Autodesk Inventor part; units mm, degrees
ref_plane "YZ Plane" through (0, 0, 0) normal (1, 0, 0) x (0, 1, 0)
ref_plane "XZ Plane" through (0, 0, 0) normal (0, 1, 0) x (-1, 0, 0)
ref_plane "XY Plane" through (0, 0, 0) normal (0, 0, 1) x (1, 0, 0)
sketch "Sketch1" plane through (0, 0, 0) normal (1, 0, 0) x (0, 1, 0)
  line L0 (-26.75, 11.75) -> (26.75, 11.75)
  line L1 (26.75, 11.75) -> (26.75, -11.75)
  line L2 (26.75, -11.75) -> (-26.75, -11.75)
  line L3 (-26.75, -11.75) -> (-26.75, 11.75)
  line L4 (-26.75, 11.75) -> (26.75, -11.75) construction
  line L5 (26.75, 11.75) -> (-26.75, -11.75) construction
  circle A0 centre (16.75, 0) radius 2.75
  circle A1 centre (-16.75, 0) radius 2.75
  point P0 (0, 0)
  dimension "d0" = 53.5
  dimension "d1" = 23.5
  dimension "d2" = 5.5
  dimension "d3" = 5.5
  dimension "d4" = 10
  dimension "d5" = 10
  dimension "d6" = 11.75
  dimension "d7" = 11.75
extrude "Extrusion1" add sketch "Sketch1" along normal blind 5
sketch "Sketch2" plane through (5, 0, 0) normal (1, 0, 0) x (0, 0, -1)
  line L0 (-11.75, 26.75) -> (-11.75, -26.75)
  line L1 (-11.75, 26.75) -> (11.75, 26.75)
  line L2 (11.75, 26.75) -> (11.75, 21.75)
  line L3 (11.75, 21.75) -> (-11.75, 21.75)
  line L4 (-11.75, 21.75) -> (-11.75, 26.75)
  line L5 (-11.75, -26.75) -> (11.75, -26.75)
  line L6 (-11.75, -26.75) -> (11.75, -26.75)
  line L7 (11.75, -26.75) -> (11.75, -21.75)
  line L8 (11.75, -21.75) -> (-11.75, -21.75)
  line L9 (-11.75, -21.75) -> (-11.75, -26.75)
  point P0 (0, 0)
  dimension "d10" = 23.5
  dimension "d11" = 5
  dimension "d12" = 23.5
  dimension "d13" = 5
extrude "Extrusion2" add sketch "Sketch2" along normal blind 15
sketch "Sketch3" plane through (0, 26.75, 11.75) normal (0, 1, 0) x (1, 0, 0)
  circle A0 centre (10, 11.75) radius 2.75
  line L0 (0, 0) -> (0, 23.5)
  line L1 (0, 0) -> (20, 0)
  point P0 (0, 11.75)
  dimension "d16" = 5.5
  dimension "d17" = 10
  dimension "d18" = 11.75
extrude "Extrusion3" cut sketch "Sketch3" against normal up to surface (53.5 mm away)
properties part number "Extrusion ends" material "Aluminum 6061"
Source: CAD feature listing. Evaluate the final solid. Frame: model axes, mm. A direction names the side the tool comes from. Round coordinates to 2 decimals unless told otherwise and drop trailing zeros. Loops run counter-clockwise (first coordinate to the right, second up) from the corner with the lowest first, then second, coordinate; pieces in that order, holes last.
1. Access query for faces 1 (the flat face through (0, 0, 0)), 2 (the flat face through (5, 0, 0)). Directions: +Z, -Z, +X, -X, +Y, -Y. A direction counts if a zero-diameter tool reaches every point of the face in a straight line with its end or side. Return the directions, or none.
2. Ray query, L1, parallel to Y at x = 13.5, z = 6.75; L2, parallel to Z at x = 10, y = -24.65; L3, parallel to X at y = 2, z = -2. Return the intervals inside material, ascending.
3. Section query B-B on y = 16.75. Output: boundary loops of the cut face in (x, z).
4. Contact query for a flat-ended pin moving along its axis: pin 1 (8 mm diameter, centred on y = 17.5, z = 0.5, fed in from +X). Output: stop coordinate, or through.
5. Mould query, pull axis Y, two halves, no side actions, for faces 3 (the flat face through (14, -21.75, 0)), 4 (the cylindrical face through (12.54, -24.22, 1.05)), 5 (the flat face through (14, 21.75, 0)), 6 (the flat face through (10, -26.75, -3)). Classes: released by +Y, released by -Y, zero draft, split by the parting line, or undercut.
6. Section query A-A on x = 14. Output: boundary loops of the cut face in (y, z), and give its area (3 significant figures).
7. Section query C-C on z = 0. Output: boundary loops of the cut face in (x, y).
8. Section query D-D on x = 10. Output: boundary loops of the cut face in (y, z), and give its area (3 significant figures).
Answers below:
1. face 1: +Z, -Z, -X, +Y, -Y
1. face 2: +Z, -Z, +X
2. L1: y = -26.75 to -21.75, 21.75 to 26.75
2. L2: z = -11.75 to -2.75, 2.75 to 11.75
2. L3: x = 0 to 5
3. outline: (0, -11.75) - (5, -11.75) - (5, -2.75) - (0, -2.75) - close; (0, 2.75) - (5, 2.75) - (5, 11.75) - (0, 11.75) - close
4. pin 1: stops at x = 5
5. face 3: undercut
5. face 4: zero draft
5. face 5: undercut
5. face 6: released by -Y
6. outline: (-26.75, -11.75) - (-21.75, -11.75) - (-21.75, 11.75) - (-26.75, 11.75) - close; (21.75, -11.75) - (26.75, -11.75) - (26.75, 11.75) - (21.75, 11.75) - close
6. area: 235 mm2
7. outline: (0, -26.75) - (7.25, -26.75) - (7.25, -21.75) - (5, -21.75) - (5, -19.5) - (0, -19.5) - close; (0, -14) - (5, -14) - (5, 14) - (0, 14) - close; (0, 19.5) - (5, 19.5) - (5, 21.75) - (7.25, 21.75) - (7.25, 26.75) - (0, 26.75) - close; (12.75, -26.75) - (20, -26.75) - (20, -21.75) - (12.75, -21.75) - close; (12.75, 21.75) - (20, 21.75) - (20, 26.75) - (12.75, 26.75) - close
8. outline: (-26.75, -11.75) - (-21.75, -11.75) - (-21.75, -2.75) - (-26.75, -2.75) - close; (-26.75, 2.75) - (-21.75, 2.75) - (-21.75, 11.75) - (-26.75, 11.75) - close; (21.75, -11.75) - (26.75, -11.75) - (26.75, -2.75) - (21.75, -2.75) - close; (21.75, 2.75) - (26.75, 2.75) - (26.75, 11.75) - (21.75, 11.75) - close
8. area: 180 mm2
